Design review of the part shown in the three views and the two pictorial views. Dimensions are in mm from the part's minimum x, y and z. A direction names the side the tool comes from. Give positions to 0.01 mm unless a question says otherwise; leave off trailing zeros. Order: outer loops, then holes, each group sorted by start corner. A loop starts at its lowest first (then second) coordinate and runs counter-clockwise, first axis right, second up.
Item 1: Consider section C-C (y = 87.5). Give the boundary of the cut face in (x, z), plus the area to 3 significant figures.
Item 2: Consider section B-B (z = 65). Give the boundary of the cut face in (x, y) (1 decimal), plus the area to 3 significant figures.
Item 3: Consider section A-A (x = 142.5). Give the boundary of the cut face in (y, z).
Item 4: For probe 1 along Z at (x, y) = (120, 79); probe 2 along X at (y, z) = (85, 14); probe 3 along Y at (x, z) = (64, 102.5), list the stretches that pass through material, from the lowest coordinate up.
Item 5: Machinability: for the marked faces 1, 2 and 3, which of the approach directions +Z, -Z, +X, -X, +Y, -Y give a long, thin tool a straight path to every point of the face, cutting with its end or side? Answer none if there is none.
Item 6: For P1, Ø3, axis at x = 139, y = 13, coming from the -Z side; P2, Ø5, axis at y = 87, z = 128, coming from the -X side; P3, Ø5, axis at x = 252, z = 88.5, coming from the +Y side, all flat-tipped, find the tip position at first contact; note any pin that passes through.
Item 7: Consider section D-D (z = 136). Give the boundary of the cut face in (x, y) (1 decimal).
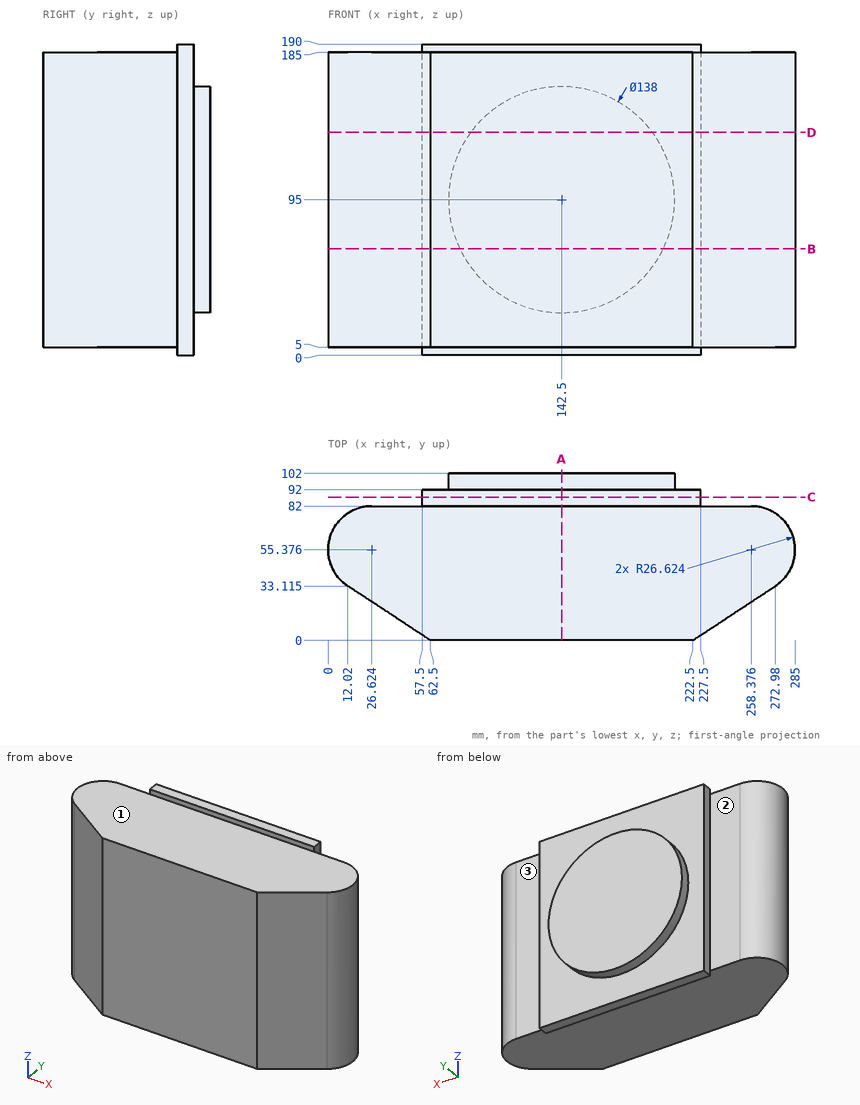
Resolved:
1. outline: (57.5, 0) - (227.5, 0) - (227.5, 190) - (57.5, 190) - close
1. area: 32,300 mm2
2. outline: (12, 33.1) - (62.5, 0) - (222.5, 0) - (273, 33.1) arc R26.6 ccw to (258.4, 82) - (227.5, 82) - (227.5, 92) - (204.6, 92) - (204.6, 102) - (80.4, 102) - (80.4, 92) - (57.5, 92) - (57.5, 82) - (26.6, 82) arc R26.6 ccw to start
2. area: 23,400 mm2
3. outline: (0, 5) - (82, 5) - (82, 0) - (92, 0) - (92, 26) - (102, 26) - (102, 164) - (92, 164) - (92, 190) - (82, 190) - (82, 185) - (0, 185) - close
4. probe 1: z = 5 to 185
4. probe 2: x = 57.5 to 227.5
4. probe 3: y = 0 to 92
5. face 1: +Z, +X, -X, -Y
5. face 2: +Z, -Z, -X, +Y
5. face 3: +Z, -Z, +X, +Y
6. P1: stops at z = 5
6. P2: stops at x = 57.5
6. P3: stops at y = 82
7. outline: (12, 33.1) - (62.5, 0) - (222.5, 0) - (273, 33.1) arc R26.6 ccw to (258.4, 82) - (227.5, 82) - (227.5, 92) - (198, 92) - (198, 102) - (87, 102) - (87, 92) - (57.5, 92) - (57.5, 82) - (26.6, 82) arc R26.6 ccw to start
